The listing builds one solid part. Answer for the finished solid, in the listing's coordinates (mm). Give positions to 0.01 mm unless a question says otherwise; leave off trailing zeros. Write each loop counter-clockwise with the first axis right and the second up, starting at its lowest first coordinate (ties: lowest second). Pieces come first, ordered by that corner, then holes.
```python
from build123d import *

# Parameters (mm, degrees)
BOSS_EXTRUDE1_DEPTH      = 51
BOSS_EXTRUDE1_DEPTH_BACK = 51
SKETCH2_R                = 4
BOSS_EXTRUDE2_DEPTH      = 10
SKETCH3_R                = 2.5
CUT_EXTRUDE1_DEPTH       = 8
SKETCH4_R                = 1.75
CUT_EXTRUDE2_DEPTH       = 30
SKETCH5_R                = 1.7
CUT_EXTRUDE3_DEPTH       = 30
SKETCH7_R                = 5
BOSS_EXTRUDE3_DEPTH      = 6.5
CUT_EXTRUDE_THIN2_DEPTH  = 2
LPATTERN1_COUNT          = 4
LPATTERN1_PITCH          = 19


with BuildPart() as part:
    # Sketch1 → Boss-Extrude1 (new, two sides: drawn at the far end of the back side and taken through both)
    with BuildSketch(Plane.XY.offset(-BOSS_EXTRUDE1_DEPTH_BACK)):
        Polygon((2.5, -4.330127019), (5, 0), (2.5, 4.330127019), (-2.5, 4.330127019), (-5, 0), (-2.5, -4.330127019), align=None)
    extrude(amount=BOSS_EXTRUDE1_DEPTH + BOSS_EXTRUDE1_DEPTH_BACK)

    # Sketch2 → Boss-Extrude2 (add)
    with BuildSketch(Plane.XY.offset(51)):
        Circle(SKETCH2_R)
    extrude(amount=BOSS_EXTRUDE2_DEPTH)

    # Sketch3 → Cut-Extrude1 (cut)
    with BuildSketch(Plane.XY.offset(61)):
        Circle(SKETCH3_R)
    extrude(amount=-CUT_EXTRUDE1_DEPTH, mode=Mode.SUBTRACT)

    # Sketch4 → Cut-Extrude2 (cut)
    with BuildSketch(Plane.XY.offset(53)):
        Circle(SKETCH4_R)
    extrude(amount=-CUT_EXTRUDE2_DEPTH, mode=Mode.SUBTRACT)

    # Sketch5 → Cut-Extrude3 (cut)
    with BuildSketch(Plane(origin=(0, 0, -51), x_dir=(-1, 0, 0), z_dir=(0, 0, -1))):
        Circle(SKETCH5_R)
    extrude(amount=-CUT_EXTRUDE3_DEPTH, mode=Mode.SUBTRACT)

    # Sketch7 → Boss-Extrude3 (add, symmetric)
    with BuildSketch(Plane.XY.offset(29.5)):
        Circle(SKETCH7_R)
    boss_extrude3 = extrude(amount=BOSS_EXTRUDE3_DEPTH, both=True)

    # Sketch8 → Cut-Extrude-Thin2 (cut, symmetric)
    with BuildSketch(Plane.XY.offset(29.5)):
        Polygon((3.366025404, -5.830127019), (-3.366025404, -5.830127019), (-6.732050808, 0), (-3.221687836, 6.080127019), (3.221687836, 6.080127019), (6.732050808, 0), align=None)
        Polygon((2.211324865, -3.830127019), (-2.211324865, -3.830127019), (-4.422649731, 0), (-2.066987298, 4.080127019), (2.066987298, 4.080127019), (4.422649731, 0), align=None, mode=Mode.SUBTRACT)
    cut_extrude_thin2 = extrude(amount=CUT_EXTRUDE_THIN2_DEPTH, both=True, mode=Mode.SUBTRACT)

    # LPattern1: Boss-Extrude3, Cut-Extrude-Thin2 ×4
    with Locations(*[(0, 0, -i * LPATTERN1_PITCH) for i in range(1, LPATTERN1_COUNT)]):
        add(boss_extrude3)
        add(cut_extrude_thin2, mode=Mode.SUBTRACT)


solid = part.part
```
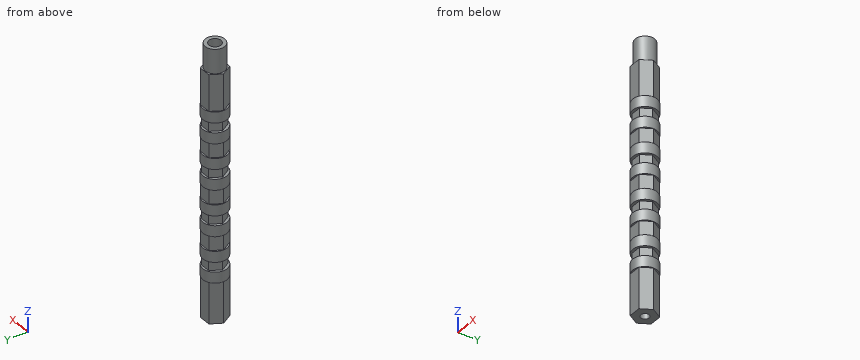
Item 1: A cutting plane is placed at A-A, the plane z = 15. Give the vertices of the cut face in (x, y), plus the area to 3 significant figures.
Conclusion:
outline: circle Ø10 at (0, 0)
area: 78.5 mm2
Item 2: Consider probe 1 along Z at (x, y) = (2.5, 3.75); probe 2 along Y at (x, z) = (0, -41.5); probe 3 along Y at (x, z) = (2.5, -43). Determine where each line is inside the solid, lowest interval first.
Conclusion:
probe 1: z = -51 to -29.5, -25.5 to -10.5, -6.5 to 8.5, 12.5 to 27.5, 31.5 to 51
probe 2: y = -4.33 to -1.7, 1.7 to 4.33
probe 3: y = -4.33 to 4.33
Item 3: Each of these flat-tipped pins is pushed along its axis until it touches: P1, Ø4, axis at y = -3, z = -22, coming from the +X side; P2, Ø0.5, axis at x = -0.5, y = -5, coming from the +Z side; P3, Ø1.2, axis at x = 0, z = 30, coming from the +Y side. Where does it stop, or does it pass through?
Conclusion:
P1: stops at x = 4.9
P2: stops at z = 36
P3: stops at y = 4.08
